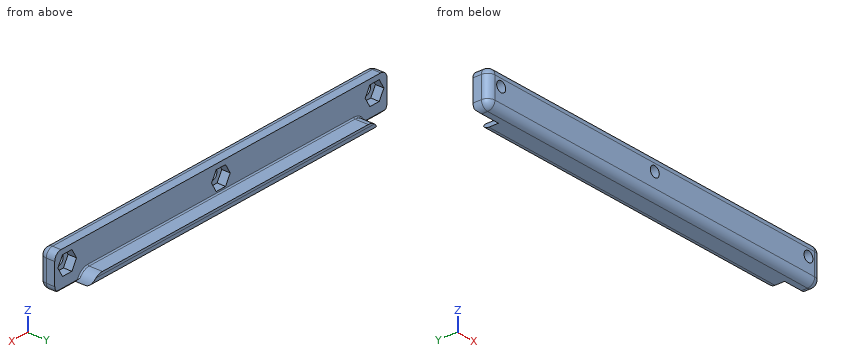
```python
from build123d import *

# Parameters (mm, degrees)
SKETCH1_W                = 160
SKETCH1_H                = 12
BOSS_EXTRUDE1_DEPTH      = 3.5
SKETCH2_W                = 160
SKETCH2_H                = 12
SKETCH2_R                = 2.15
BOSS_EXTRUDE2_DEPTH      = 3
BOSS_EXTRUDE3_DEPTH      = 6
BOSS_EXTRUDE3_DEPTH_BACK = 6.5
CAVITY1_START            = 2.5
CAVITY1_DEPTH            = 7.5
CAVITY1_START_2          = -160
CAVITY1_2_DEPTH          = 160
FILLET2_R                = 3
FILLET3_R                = 3
FILLET4_R                = 0.5


with BuildPart() as part:
    # Sketch1 → Boss-Extrude1 (new body)
    with BuildSketch(Plane(origin=(0, 0, 0), x_dir=(1, 0, 0), z_dir=(0, 1, 0))):
        with Locations((-80, -6)):
            Rectangle(SKETCH1_W, SKETCH1_H)
        Polygon((-75.5, -6), (-77.75, -2.102885683), (-82.25, -2.102885683), (-84.5, -6), (-82.25, -9.897114317), (-77.75, -9.897114317), align=None, mode=Mode.SUBTRACT)
        Polygon((-149.5, -6), (-151.75, -2.102885683), (-156.25, -2.102885683), (-158.5, -6), (-156.25, -9.897114317), (-151.75, -9.897114317), align=None, mode=Mode.SUBTRACT)
        Polygon((-10.5, -6), (-8.25, -9.897114317), (-3.75, -9.897114317), (-1.5, -6), (-3.75, -2.102885683), (-8.25, -2.102885683), align=None, mode=Mode.SUBTRACT)
    extrude(amount=BOSS_EXTRUDE1_DEPTH)

    # Sketch2 → Boss-Extrude2 (add)
    with BuildSketch(Plane.XZ):
        with Locations((-80, 6)):
            Rectangle(SKETCH2_W, SKETCH2_H)
        with Locations(Location((-154, 6, 0), (0, 0, 270))):
            Circle(SKETCH2_R, mode=Mode.SUBTRACT)
        with Locations(Location((-80, 6, 0), (0, 0, 270))):
            Circle(SKETCH2_R, mode=Mode.SUBTRACT)
        with Locations(Location((-6, 6, 0), (0, 0, 270))):
            Circle(SKETCH2_R, mode=Mode.SUBTRACT)
    extrude(amount=BOSS_EXTRUDE2_DEPTH)

    # Sketch3 → Boss-Extrude3 (add, two sides: drawn at the far end of the back side and taken through both)
    with BuildSketch(Plane(origin=(0, 3.5, 0), x_dir=(1, 0, 0), z_dir=(0, 1, 0)).offset(-BOSS_EXTRUDE3_DEPTH_BACK)):
        Polygon((-80, -1), (0, -1), (0, 3), (-160, 3), (-160, -1), align=None)
    extrude(amount=BOSS_EXTRUDE3_DEPTH + BOSS_EXTRUDE3_DEPTH_BACK)

    # Cavity1: read off the stored shape, not the designer's step
    # Cavity1 outline → Cavity1 (cut)
    with BuildSketch(Plane(origin=(0, 0, 0), x_dir=(1, 0, 0), z_dir=(0, 1, 0)).offset(CAVITY1_START)):
        with BuildLine():
            ThreePointArc((-11.101020514, 3), (-12.83772234, 0.127016654), (-16, -1))
            Line((-16, -1), (0, -1))
            Line((0, -1), (0, 3))
            Line((0, 3), (-11.101020514, 3))
        make_face()
        with BuildLine():
            Line((-160, -1), (-144, -1))
            ThreePointArc((-144, -1), (-147.16227766, 0.127016654), (-148.898979486, 3))
            Line((-148.898979486, 3), (-160, 3))
            Line((-160, 3), (-160, -1))
        make_face()
    extrude(amount=CAVITY1_DEPTH, mode=Mode.SUBTRACT)

    # Cavity1 2 outline → Cavity1 2 (add)
    with BuildSketch(Plane.YZ.offset(CAVITY1_START_2)):
        Polygon((2.5, -3), (3.5, -2), (3.5, 1), (2.5, 1), align=None)
    extrude(amount=CAVITY1_2_DEPTH)

    # Fillet2
    fillet2_edges = [part.edges().sort_by_distance(p)[0] for p in [
        (-80, 9.5, -3),
    ]]
    fillet(fillet2_edges, radius=FILLET2_R)

    # Fillet3
    fillet3_edges = [part.edges().sort_by_distance(p)[0] for p in [
        (-80, -3, 12),
        (0, -3, 4.5),
        (-160, -3, 4.5),
        (-160, -0.25, -3),
        (-80, -3, -3),
        (0, -0.25, -3),
        (-160, 0.25, 12),
        (0, 0.25, 12),
    ]]
    fillet(fillet3_edges, radius=FILLET3_R)

    # Fillet4
    fillet4_edges = [part.edges().sort_by_distance(p)[0] for p in [
        (-80, 3.5, 1),
        (-146.738612787, 3.5, 0.183300132),
        (-13.261387213, 3.5, 0.183300132),
    ]]
    fillet(fillet4_edges, radius=FILLET4_R)


solid = part.part
```
Check sheet for the modelled part. Datum: model origin and axes. Units: mm. Coordinates: 2 decimals unless noted, no trailing zeros. Write each loop counter-clockwise with the first axis right and the second up, starting at its lowest first coordinate (ties: lowest second). Pieces come first, ordered by that corner, then holes. Notation, with made-up numbers: M 55.25,85.5 L 104.25,85.5 A6 ccw 104.25,89.5 Z; hole C 25.25,14 d6. An arc over 180 degrees is marked long. Use one line per item in the form item = value.
Item 1: Sectioned sample at B-B, the plane x = -120. Record the cut outline in (y, z), and give its area (3 significant figures).
Answer below:
outline = M -3,0 A3 ccw 0,-3 L 6.5,-3 A3 ccw 9.5,0 L 9.5,1 L 4,1 A0.5 cw 3.5,1.5 L 3.5,12 L 0,12 A3 ccw -3,9 Z
area = 116 mm^2
Item 2: Material ranges on L1, parallel to X at y = -1.7, z = 6; L2, parallel to X at y = 1, z = 7.25; L3, parallel to Y at x = -131.5, z = 7, recorded low to high. Write a range as from..to.
Answer below:
L1 = -159.47..-156.15, -151.85..-82.15, -77.85..-8.15, -3.85..-0.53
L2 = -160..-157.78, -150.22..-83.78, -76.22..-9.78, -2.22..0
L3 = -3..3.5
Item 3: Sectioned sample at C-C, the plane x = -80. Record the cut outline in (y, z), and give its area (3 significant figures).
Answer below:
outline = M -3,0 A3 ccw 0,-3 L 6.5,-3 A3 ccw 9.5,0 L 9.5,1 L 4,1 A0.5 cw 3.5,1.5 L 3.5,2.1 L 0,2.1 L 0,3.85 L -3,3.85 Z; M -3,8.15 L 0,8.15 L 0,9.9 L 3.5,9.9 L 3.5,12 L 0,12 A3 ccw -3,9 Z
area = 75.6 mm^2
Item 4: Gauge pin test, flat ends, axial feed: pin 1 Ø8.5 at (x, z) = (-152, 4) entering from +Y; pin 2 Ø4 at (x, z) = (-92.5, 9.5) entering from -Y; pin 3 Ø6 at (x, z) = (-79.5, 6) entering from +Y; pin 4 Ø3 at (x, y) = (-62, 7) entering from +Z. Record the tip position at first contact, or that the pin passes through.
Answer below:
pin_1 = 3.5
pin_2 = -3
pin_3 = 0
pin_4 = 1
Item 5: Sectioned sample at A-A, the plane x = -154. Record the cut outline in (y, z), and give its area (3 significant figures).
Answer below:
outline = M -3,0 A3 ccw 0,-3 L 2.5,-3 L 3.5,-2 L 3.5,2.1 L 0,2.1 L 0,3.85 L -3,3.85 Z; M -3,8.15 L 0,8.15 L 0,9.9 L 3.5,9.9 L 3.5,12 L 0,12 A3 ccw -3,9 Z
area = 53.0 mm^2
